```python
from build123d import *

# Parameters (mm, degrees)
EXTRUDE_1_DEPTH     = 12.7
SKETCH_2_R          = 4.3053
CUT_EXTRUDE_1_DEPTH = 184.601770144
CUT_EXTRUDE_2_DEPTH = 184.601770144
SKETCH_4_R          = 10.3124
CUT_EXTRUDE_3_DEPTH = 7.9502
SKETCH_5_R          = 6.7437
CUT_EXTRUDE_4_DEPTH = 184.601770144
SKETCH_6_R          = 9.525
CUT_EXTRUDE_5_DEPTH = 5.244874679
CUT_EXTRUDE_5_DRAFT = -41
SKETCH_7_R          = 4.9657
CUT_EXTRUDE_6_DEPTH = 184.601770144
SKETCH_8_R          = 2.0193
CUT_EXTRUDE_7_DEPTH = 9.525
CHAMFER_1_SIZE      = 0.762


with BuildPart() as part:
    # 草图1 → 凸台-拉伸1 (new body)
    with BuildSketch(Plane.XY):
        with BuildLine():
            Line((6.35, 0), (146.05, 0))
            ThreePointArc((146.05, 0), (150.540128061, 1.859871939), (152.4, 6.35))
            Line((152.4, 6.35), (152.4, 95.25))
            ThreePointArc((152.4, 95.25), (150.540128061, 99.740128061), (146.05, 101.6))
            Line((146.05, 101.6), (6.35, 101.6))
            ThreePointArc((6.35, 101.6), (1.859871939, 99.740128061), (0, 95.25))
            Line((0, 95.25), (0, 6.35))
            ThreePointArc((0, 6.35), (1.859871939, 1.859871939), (6.35, 0))
        make_face()
    extrude(amount=EXTRUDE_1_DEPTH)

    # 草图2 → 切除-拉伸1 (cut, through all)
    with BuildSketch(Plane.XY.offset(12.7)):
        with Locations((9.525, 9.525)):
            Circle(SKETCH_2_R)
        with Locations((142.875, 9.525)):
            Circle(SKETCH_2_R)
        with Locations((9.525, 92.075)):
            Circle(SKETCH_2_R)
        with Locations((142.875, 92.075)):
            Circle(SKETCH_2_R)
    extrude(amount=-CUT_EXTRUDE_1_DEPTH, mode=Mode.SUBTRACT)

    # 草图3 → 切除-拉伸2 (cut, through all)
    with BuildSketch(Plane.XY.offset(12.7)):
        with BuildLine():
            Line((63.5, 15.875), (88.9, 15.875))
            ThreePointArc((88.9, 15.875), (92.075, 19.05), (88.9, 22.225))
            Line((88.9, 22.225), (63.5, 22.225))
            ThreePointArc((63.5, 22.225), (60.325, 19.05), (63.5, 15.875))
        make_face()
    extrude(amount=-CUT_EXTRUDE_2_DEPTH, mode=Mode.SUBTRACT)

    # 草图4 → 切除-拉伸3 (cut)
    with BuildSketch(Plane.XY.offset(12.7)):
        with Locations((38.1, 50.8)):
            Circle(SKETCH_4_R)
    extrude(amount=-CUT_EXTRUDE_3_DEPTH, mode=Mode.SUBTRACT)

    # 草图5 → 切除-拉伸4 (cut, through all)
    with BuildSketch(Plane.XY.offset(12.7)):
        with Locations((38.1, 50.8)):
            Circle(SKETCH_5_R)
    extrude(amount=-CUT_EXTRUDE_4_DEPTH, mode=Mode.SUBTRACT)


with BuildPart() as cut_extrude_5_tool:
    # 草图6 → 切除-拉伸5 (with draft: the straight prism first)
    with BuildSketch(Plane.XY.offset(12.7)):
        with Locations((114.3, 50.8)):
            Circle(SKETCH_6_R)
    extrude(amount=-CUT_EXTRUDE_5_DEPTH)
    # 切除-拉伸5: the draft: its side faces are tilted about the plane it starts from
    cut_extrude_5_sides = [cut_extrude_5_tool.faces().sort_by_distance(p)[0] for p in [
        (104.775, 50.8, 10.07756266),
    ]]
    draft(cut_extrude_5_sides, Plane.XY.offset(12.7), CUT_EXTRUDE_5_DRAFT)


with BuildPart() as part_1:
    add(part.part)

    # 切除-拉伸5: cut by cut_extrude_5_tool
    add(cut_extrude_5_tool.part, mode=Mode.SUBTRACT)

    # 草图7 → 切除-拉伸6 (cut, through all)
    with BuildSketch(Plane.XY.offset(12.7)):
        with Locations((114.3, 50.8)):
            Circle(SKETCH_7_R)
    extrude(amount=-CUT_EXTRUDE_6_DEPTH, mode=Mode.SUBTRACT)

    # 草图8 → 切除-拉伸7 (cut)
    with BuildSketch(Plane.XY.offset(12.7)):
        with Locations((114.3, 66.675)):
            Circle(SKETCH_8_R)
        with Locations((97.802, 42.725)):
            Circle(SKETCH_8_R)
        with Locations((130.798, 42.725)):
            Circle(SKETCH_8_R)
    extrude(amount=-CUT_EXTRUDE_7_DEPTH, mode=Mode.SUBTRACT)

    # 倒角1
    chamfer_1_edges = [part_1.edges().sort_by_distance(p)[0] for p in [
        (150.540128061, 1.859871939, 12.7),
        (152.4, 50.8, 12.7),
        (150.540128061, 99.740128061, 12.7),
        (76.2, 101.6, 12.7),
        (1.859871939, 99.740128061, 12.7),
        (0, 50.8, 12.7),
        (1.859871939, 1.859871939, 12.7),
        (76.2, 0, 12.7),
    ]]
    chamfer(chamfer_1_edges, length=CHAMFER_1_SIZE)


solid = part_1.part
```
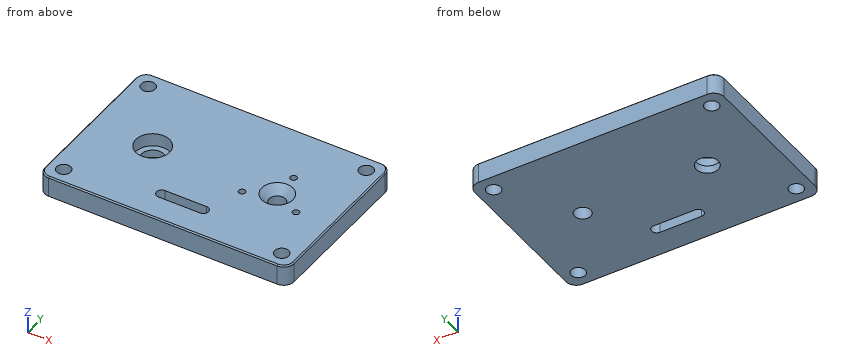
Work out the finished part from the listing and answer in its coordinate system (mm). Round coordinates to 2 decimals unless told otherwise and drop trailing zeros. Write each loop counter-clockwise with the first axis right and the second up, starting at its lowest first coordinate (ties: lowest second). Pieces come first, ordered by that corner, then holes. Notation, with made-up numbers: (50.5, -10.5) - (72.5, -10.5) arc R31 cw to (72.5, 28.5) - close; hole circle Ø3 at (-16, 49.5). An arc over 180 degrees is marked (long way). Return JSON: item names as keys, results as strings. Group by question number.
Q1. The part is cut by section C-C on y = 19.05. Write down the section's boundary in (x, z) (3 decimals), then the cut area to 3 significant figures.
Q2. The part is cut by section B-B on y = 50.8. Write down the section's boundary in (x, z) (3 decimals), then the cut area to 3 significant figures.
Q3. Each of these flat-tipped pins is pushed along its axis until it touches: pin 1 Ø1.2 at (x, y) = (97.5, 42.5) entering from +Z (3 decimals); pin 2 Ø6 at (x, y) = (35, 46.5) entering from +Z; pin 3 Ø5 at (x, y) = (142.875, 9.525) entering from +Z. Where does it stop, or does it pass through?
Q4. The part is cut by section D-D on x = 143. Write down the section's boundary in (y, z).
Q5. Find the intervals of material crossed by L1, parallel to Y at x = 9.5, z = 6.5; L2, parallel to X at y = 51.5, z = 3; L3, parallel to Y at x = 114.3, z = 7.5, in increasing order.
Q6. The part is cut by section A-A on x = 38.1. Write down the section's boundary in (y, z), then the cut area to 3 significant figures.
Solved:
{
 "1": {"outline": "(0, 0) - (60.325, 0) - (60.325, 12.7) - (0.762, 12.7) - (0, 11.938) - close; (92.075, 0) - (152.4, 0) - (152.4, 11.938) - (151.638, 12.7) - (92.075, 12.7) - close", "area": "1,530 mm²"},
 "2": {"outline": "(0, 0) - (31.356, 0) - (31.356, 4.75) - (27.788, 4.75) - (27.788, 12.7) - (0.762, 12.7) - (0, 11.938) - close; (44.844, 0) - (109.334, 0) - (109.334, 7.455) - (104.775, 12.7) - (48.412, 12.7) - (48.412, 4.75) - (44.844, 4.75) - close; (119.266, 0) - (152.4, 0) - (152.4, 11.938) - (151.638, 12.7) - (123.825, 12.7) - (119.266, 7.455) - close", "area": "1,560 mm²"},
 "3": {"pin 1": "z = 3.175", "pin 2": "z = 4.75", "pin 3": "through"},
 "4": {"outline": "(0, 0) - (5.22, 0) - (5.22, 12.7) - (0.76, 12.7) - (0, 11.94) - close; (13.83, 0) - (87.77, 0) - (87.77, 12.7) - (13.83, 12.7) - close; (96.38, 0) - (101.6, 0) - (101.6, 11.94) - (100.84, 12.7) - (96.38, 12.7) - close"},
 "5": {"L1": "0 to 5.22, 13.83 to 87.77, 96.38 to 101.6", "L2": "0 to 31.39, 44.81 to 109.38, 119.22 to 152.4", "L3": "0 to 45.8, 55.8 to 64.66, 68.69 to 101.6"},
 "6": {"outline": "(0, 0) - (44.06, 0) - (44.06, 4.75) - (40.49, 4.75) - (40.49, 12.7) - (0.76, 12.7) - (0, 11.94) - close; (57.54, 0) - (101.6, 0) - (101.6, 11.94) - (100.84, 12.7) - (61.11, 12.7) - (61.11, 4.75) - (57.54, 4.75) - close", "area": "1,060 mm²"}
}
